Geometry check sheet. Reference: the model listing, model coordinates, mm. Face numbers are marked on the shaded views. Round coordinates to 2 decimals unless told otherwise and drop trailing zeros. Loops run counter-clockwise (first coordinate to the right, second up) from the corner with the lowest first, then second, coordinate; pieces in that order, holes last. Notation, with made-up numbers: M -32.5,-35.75 L -5.5,-35.75 A17 ccw -5.5,-21.75 Z; hole C 44.5,-9.75 d10. An arc over 180 degrees is marked long. Use one line per item in the form item = value. Start each with the question number.
1. Draft check along Y on the marked faces 1, 2, 3 and 4. Enter one of: pulls with the +Y half, pulls with the -Y half, needs draft (parallel to the pull), parting line crosses it, or undercut.
2. Material ranges on line 1 (Y direction, x = 5, z = -4.5); line 2 (Z direction, x = 16.5, y = 12.5); line 3 (Y direction, x = 11, z = 3.5), recorded low to high.
3. Cross-section at B-B (z = -5). Record the boundary of the cut face in (x, y).
4. Cross-section at D-D (x = -8.5). Record the boundary of the cut face in (y, z).
5. Go/stop test with flat-tipped pins: pin 1 (2 mm diameter, centred on x = -7.5, y = 3.5, fed in from +Z); pin 2 (4 mm diameter, centred on y = 10.33, z = -15.05, fed in from -X); pin 3 (4 mm diameter, centred on x = 5.5, y = 1.5, fed in from -Z); pin 4 (12 mm diameter, centred on x = 14.5, y = 23.5, fed in from -Z). Record where each tip stops, or that it passes through.
6. Cross-section at C-C (z = 13.5). Record the boundary of the cut face in (x, y).
7. Cross-section at A-A (x = 5). Record the boundary of the cut face in (y, z), then the cut area to 3 significant figures.
```python
from build123d import *
from build123d.topology import SkipClean

# Parameters (mm, degrees)
BOSS_EXTRUDE1_DEPTH     = 4
SKETCH3_W               = 5
SKETCH3_H               = 30
BOSS_EXTRUDE3_DEPTH     = 24
BOSS_EXTRUDE5_DEPTH     = 5
SKETCH7_3_R             = 3.25755
CUT_EXTRUDE3_DEPTH      = 5
FILLET3_R               = 10
BOSS_EXTRUDE8_START     = -4
BOSS_EXTRUDE8_DEPTH     = 4
BOSS_EXTRUDE9_DEPTH     = 4
CUT_EXTRUDE4_DEPTH      = 25
CUT_EXTRUDE4_DEPTH_BACK = 1
SKETCH8_R               = 7.5
CUT_EXTRUDE5_DEPTH      = 50.517048882
CUT_EXTRUDE5_DEPTH_BACK = 50.517048882
SKETCH9_R               = 2.75
FILLET4_R               = 1
BOSS_EXTRUDE6_START     = -4
BOSS_EXTRUDE6_DEPTH     = 4
FILLET6_R               = 2
BOSS_EXTRUDE7_DEPTH     = 4


# Read off the part's stored shape, not the designer's step: Boss-Extrude8
with BuildPart() as part:
    # Sketch2 → Boss-Extrude1 (new body)
    with BuildSketch(Plane(origin=(0, 0, 0), x_dir=(1, 0, 0), z_dir=(0, 1, 0))):
        with BuildLine():
            Line((18.000912404, -14.946929254), (18.000912404, 15.053070746))
            Line((18.000912404, 15.053070746), (0.039090451, 15.053070746))
            ThreePointArc((0.039090451, 15.053070746), (-10.199781301, 11.024824414), (-14.94907539, 1.099832277))
            Line((-14.94907539, 1.099832277), (-5.983249792, 0.448020006))
            ThreePointArc((-5.983249792, 0.448020006), (3.000957071, 5.20912276), (3.369824569, -4.951979994))
            Line((3.369824569, -4.951979994), (10.151696986, -14.946929254))
            Line((10.151696986, -14.946929254), (18.000912404, -14.946929254))
        make_face()
    boss_extrude1 = extrude(amount=BOSS_EXTRUDE1_DEPTH)

    # Sketch3 → Boss-Extrude3 (add)
    with BuildSketch(Plane(origin=(0, 4, 0), x_dir=(1, 0, 0), z_dir=(0, 1, 0))):
        with Locations((15.500912404, 0.053070746)):
            Rectangle(SKETCH3_W, SKETCH3_H)
    extrude(amount=BOSS_EXTRUDE3_DEPTH)

    # Mirror1: Boss-Extrude1 across plane
    add(boss_extrude1.mirror(Plane.ZX.offset(16)))

    # Sketch7 → Boss-Extrude5 (add)
    with BuildSketch(Plane.ZY.offset(-13.000912404)):
        with BuildLine():
            Line((-15.053070746, 0), (-15.053070746, 4))
            Line((-15.053070746, 4), (-15.053070746, 7.075913265))
            ThreePointArc((-15.053070746, 7.075913265), (-18.310620746, 10.333463265), (-15.053070746, 13.591013265))
            Line((-15.053070746, 13.591013265), (-15.053070746, 20.666926531))
            ThreePointArc((-15.053070746, 20.666926531), (-25.386534011, 10.333463265), (-15.053070746, 0))
        make_face()
        with BuildLine():
            ThreePointArc((25.146929254, 21.8), (22.159418422, 29.012489168), (14.946929254, 32))
            Line((14.946929254, 32), (14.946929254, 28))
            Line((14.946929254, 28), (14.946929254, 25.05755))
            ThreePointArc((14.946929254, 25.05755), (17.250364949, 24.103435695), (18.204479254, 21.8))
            ThreePointArc((18.204479254, 21.8), (17.250364949, 19.496564305), (14.946929254, 18.54245))
            Line((14.946929254, 18.54245), (14.946929254, 11.6))
            ThreePointArc((14.946929254, 11.6), (22.159418422, 14.587510832), (25.146929254, 21.8))
        make_face()
        with BuildLine():
            Line((14.946929254, 28), (14.946929254, 32))
            ThreePointArc((14.946929254, 32), (4.746929254, 21.8), (14.946929254, 11.6))
            Line((14.946929254, 11.6), (14.946929254, 18.54245))
            ThreePointArc((14.946929254, 18.54245), (11.689379254, 21.8), (14.946929254, 25.05755))
            Line((14.946929254, 25.05755), (14.946929254, 28))
        make_face()
    extrude(amount=-BOSS_EXTRUDE5_DEPTH)

    # Sketch7<3> → Cut-Extrude3 (cut)
    with SkipClean():  # the faces are left unmerged after this step: merging them gives an invalid solid
        with BuildSketch(Plane.ZY.offset(-13.000912404)):
            with Locations((14.946929254, 21.8)):
                Circle(SKETCH7_3_R)
            with Locations((-15.053070746, 10.333463265)):
                Circle(SKETCH7_3_R)
        extrude(amount=-CUT_EXTRUDE3_DEPTH, mode=Mode.SUBTRACT)

    # Fillet3
    # the kernel refuses this fillet: 10 mm, written as the material it adds along each edge
    with BuildSketch(Plane(origin=(13.000912404, 20.666926531, -15.053070746), x_dir=(0, -0.25425566101904284, -0.9671370424297528), z_dir=(1, 0, 0))) as fillet3_piece_1:
        with BuildLine():
            CenterArc((7.797239676, 9.671370424), FILLET3_R, 194.729484057, 60.541031886)
            Line((-1.874130748, 7.128813814), (0, 0))
            ThreePointArc((0, 0), (2.627341533, 0.339588165), (5.254683066, 0))
        make_face()
    extrude(amount=5)
    with BuildSketch(Plane(origin=(13.000912404, 11.6, 14.946929254), x_dir=(0, -1, 0), z_dir=(1, 0, 0))) as fillet3_piece_2:
        with BuildLine():
            CenterArc((7.351068344, -10), FILLET3_R, 90, 60.326985198)
            ThreePointArc((-1.337579351, -5.04950495), (-0.340063626, -2.611829759), (0, 0))
            Line((0, 0), (7.351068344, 0))
        make_face()
    extrude(amount=5)

    # Boss-Extrude8 outline → Boss-Extrude8 (add)
    with SkipClean():  # the faces are left unmerged after this step: merging them gives an invalid solid
        with BuildSketch(Plane.XZ.offset(BOSS_EXTRUDE8_START)):
            with BuildLine():
                ThreePointArc((-5.983249792, -0.448020006), (-3.002134964, 5.194919216), (3.375546051, 4.960412166))
                Line((3.375546051, 4.960412166), (10.151696986, 14.946929254))
                Line((10.151696986, 14.946929254), (0, 14.989479178))
                ThreePointArc((0, 14.989479178), (-10.981129247, 10.202905787), (-14.94907539, -1.099832277))
                Line((-14.94907539, -1.099832277), (-5.983249792, -0.448020006))
            make_face()
        extrude(amount=BOSS_EXTRUDE8_DEPTH)

    # Sketch13 → Boss-Extrude9 (add)
    with SkipClean():  # the faces are left unmerged after this step: merging them gives an invalid solid
        with BuildSketch(Plane(origin=(0, 32, 0), x_dir=(1, 0, 0), z_dir=(0, 1, 0))):
            with BuildLine():
                Line((10.151696986, -14.946929254), (8.443727077, -12.429767101))
                ThreePointArc((8.443727077, -12.429767101), (4.471376939, -14.331468239), (0.118292185, -14.999813933))
                Line((0.118292185, -14.999813933), (10.151696986, -14.946929254))
            make_face()
            with BuildLine():
                ThreePointArc((6.07616266, 0.026524042), (5.364215569, -2.817642503), (3.396292996, -4.990988482))
                Line((3.396292996, -4.990988482), (8.443727077, -12.429767101))
                ThreePointArc((8.443727077, -12.429767101), (13.307281184, -7.027001355), (15.065637155, 0.026524042))
                ThreePointArc((15.065637155, 0.026524042), (10.664463523, 10.651897114), (0.039090451, 15.053070746))
                ThreePointArc((0.039090451, 15.053070746), (-10.199781301, 11.024824414), (-14.94907539, 1.099832277))
                Line((-14.94907539, 1.099832277), (-5.983249792, 0.448020006))
                ThreePointArc((-5.983249792, 0.448020006), (0.249967121, 6.059912135), (6.07616266, 0.026524042))
            make_face()
            with BuildLine():
                Line((8.443727077, -12.429767101), (3.396292996, -4.990988482))
                ThreePointArc((3.396292996, -4.990988482), (-2.989348597, -5.196003869), (-5.983249792, 0.448020006))
                Line((-5.983249792, 0.448020006), (-14.94907539, 1.099832277))
                ThreePointArc((-14.94907539, 1.099832277), (-10.932188175, -10.241297106), (0.118292185, -14.999813933))
                ThreePointArc((0.118292185, -14.999813933), (4.471376939, -14.331468239), (8.443727077, -12.429767101))
            make_face()
        extrude(amount=-BOSS_EXTRUDE9_DEPTH)

    # Sketch8 → Cut-Extrude4 (cut, two sides: drawn at the far end of the back side and taken through both)
    with SkipClean():  # the faces are left unmerged after this step: merging them gives an invalid solid
        with BuildSketch(Plane(origin=(0, 4, 0), x_dir=(1, 0, 0), z_dir=(0, 1, 0)).offset(-CUT_EXTRUDE4_DEPTH_BACK)):
            with Locations(Location((0, 0, 0), (0, 0, 90))):
                Circle(SKETCH8_R)
        extrude(amount=CUT_EXTRUDE4_DEPTH + CUT_EXTRUDE4_DEPTH_BACK, mode=Mode.SUBTRACT)

    # Sketch9 → Cut-Extrude5 (cut, two sides: drawn at the far end of the back side and taken through both)
    with BuildSketch(Plane.ZY.offset(-13.000912404).offset(-CUT_EXTRUDE5_DEPTH_BACK)):
        with Locations((9, 10.2)):
            Circle(SKETCH9_R)
        with Locations((-9, 21.8)):
            Circle(SKETCH9_R)
    extrude(amount=CUT_EXTRUDE5_DEPTH + CUT_EXTRUDE5_DEPTH_BACK, mode=Mode.SUBTRACT)

    # Fillet4
    fillet4_edges = [part.edges().sort_by_distance(p)[0] for p in [
        (13.000912404, 4, -0.053070746),
        (13.000912404, 28, -0.053070746),
    ]]
    fillet(fillet4_edges, radius=FILLET4_R)

    # Sketch10 → Boss-Extrude6 (add)
    with BuildSketch(Plane.XZ.offset(BOSS_EXTRUDE6_START)):
        with BuildLine():
            ThreePointArc((0.039090451, -15.053070746), (-5.733491903, -13.900038334), (-10.620178824, -10.617892431))
            Line((-10.620178824, -10.617892431), (-9.005905934, -15.053070746))
            Line((-9.005905934, -15.053070746), (0.039090451, -15.053070746))
        make_face()
    extrude(amount=BOSS_EXTRUDE6_DEPTH)

    # Fillet6
    fillet6_edges = [part.edges().sort_by_distance(p)[0] for p in [
        (-9.005905934, 2, -15.053070746),
    ]]
    fillet(fillet6_edges, radius=FILLET6_R)

    # Sketch11 → Boss-Extrude7 (add)
    with BuildSketch(Plane(origin=(0, 32, 0), x_dir=(1, 0, 0), z_dir=(0, 1, 0))):
        with BuildLine():
            Line((-9.484876099, 13.737111032), (-10.620178824, 10.617892431))
            ThreePointArc((-10.620178824, 10.617892431), (-5.733491903, 13.900038334), (0.039090451, 15.053070746))
            Line((0.039090451, 15.053070746), (-7.605490857, 15.053070746))
            ThreePointArc((-7.605490857, 15.053070746), (-8.75264373, 14.691374834), (-9.484876099, 13.737111032))
        make_face()
    extrude(amount=-BOSS_EXTRUDE7_DEPTH)


solid = part.part
```
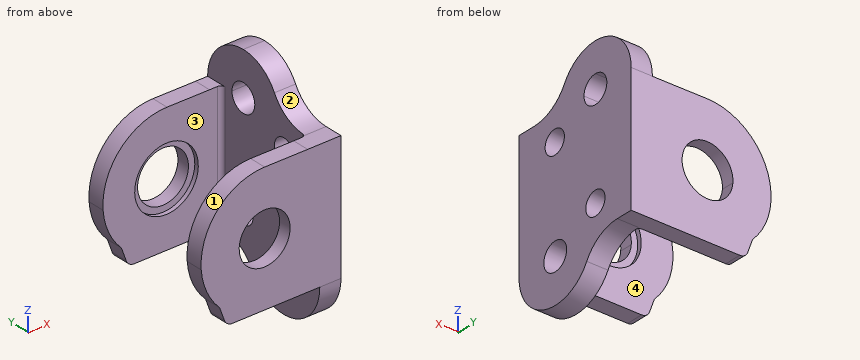
Reported:
q1.face_1 = needs draft
q1.face_2 = pulls with the -Y half
q1.face_3 = undercut
q1.face_4 = undercut
q2.line_1 = 0 to 3, 29 to 32
q2.line_2 = -25.16 to -17.49, -12.62 to 7.49, 10.51 to 19.3
q2.line_3 = 0 to 4, 28 to 32
q3.outline = M -14.14,0 L -3.34,0 L -3.34,3 L -5.59,3 L -5.59,4 L -14.14,4 Z; M -14.14,28 L -5.59,28 L -5.59,29 L -3.34,29 L -3.34,32 L -14.14,32 Z; M 3.34,0 L 18,0 L 18,32 L 3.34,32 L 3.34,29 L 5.59,29 L 5.59,28 L 12,28 A1 cw 13,27 L 13,5 A1 cw 12,4 L 5.59,4 L 5.59,3 L 3.34,3 Z
q4.outline = M 0,-14.84 L 4,-14.84 L 4,12.35 L 0,12.35 Z; M 28,-14.84 L 32,-14.84 L 32,12.34 L 28,12.34 Z
q5.pin_1 = 13.51
q5.pin_2 = through
q5.pin_3 = -15.05
q5.pin_4 = -22.5
q6.outline = M -6.51,0 L 18,0 L 18,18.88 L 13,18.88 L 13,5 A1 cw 12,4 L -6.51,4 Z; M -6.51,28 L 12,28 A1 cw 13,27 L 13,24.72 L 18,24.72 L 18,32 L -6.51,32 Z
q7.outline = M 0,-15.05 L 4,-15.05 L 4,-5.59 L 3,-5.59 L 3,-3.33 L 0,-3.33 Z; M 0,3.31 L 3,3.31 L 3,5.59 L 4,5.59 L 4,14.97 L 0,14.97 Z; M 28,-15.05 L 32,-15.05 L 32,-3.33 L 29,-3.33 L 29,-5.59 L 28,-5.59 Z; M 28,5.59 L 29,5.59 L 29,3.31 L 32,3.31 L 32,14.97 L 28,14.97 Z
q7.area = 178 mm²
